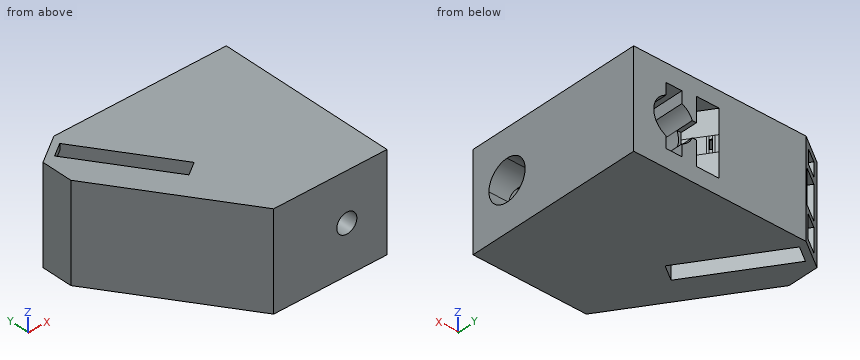
```python
from build123d import *
from build123d.topology import SkipClean

# Parameters (mm, degrees)
BOSS_EXTRUDE1_DEPTH     = 2.5
BOSS_EXTRUDE1_2_DEPTH   = 2.5
BOSS_EXTRUDE2_DEPTH     = 6.35
BOSS_EXTRUDE3_DEPTH     = 6.35
SKETCH4_R               = 3.175
CUT_EXTRUDE1_DEPTH      = 25.4
SKETCH5_R               = 1.5875
CUT_EXTRUDE2_DEPTH      = 25.4
CUT_EXTRUDE3_DEPTH      = 25.4
CUT_EXTRUDE4_REACH      = 43
CUT_EXTRUDE4_END_RADIUS = 3.175
CUT_EXTRUDE5_REACH      = 39.36
SKETCH8_W               = 2.54
SKETCH8_H               = 9.525
SKETCH9_W               = 0.508
SKETCH9_H               = 15.2
BOSS_EXTRUDE4_DEPTH     = 17
BOSS_EXTRUDE5_DEPTH     = 1.016
SKETCH11_W              = 1.176658287
SKETCH11_H              = 2.5
SKETCH11_W_2            = 2.433787944
SKETCH11_H_2            = 15.2
BOSS_EXTRUDE6_DEPTH     = 1.27
CUT_EXTRUDE6_DEPTH      = 38.864332241
BOSS_EXTRUDE7_START     = 2.54
BOSS_EXTRUDE7_DEPTH     = 2.54
BOSS_EXTRUDE8_DEPTH     = 2.54
BOSS_EXTRUDE9_DEPTH     = 0.508
BOSS_EXTRUDE10_DEPTH    = 0.508
CUT_EXTRUDE7_DEPTH      = 3.81
CUT_EXTRUDE8_DEPTH      = 3.81
BOSS_EXTRUDE11_DEPTH    = 3.81
SKETCH21_W              = 1.016
SKETCH21_H              = 1.016
SKETCH21_W_2            = 0.889
BOSS_EXTRUDE12_DEPTH    = 3.302
BOSS_EXTRUDE13_DEPTH    = 3.81


with BuildPart() as part:
    # Sketch1 → Boss-Extrude1 (new body)
    with BuildSketch(Plane.XY):
        Polygon((5.08, 0), (0, 0), (0, 19.141079028), (-1.033059908, 19.141079028), (-3.75575709, 23.125698967), (-8.376397661, 9.077684872), (-11.679025045, 6.820994294), (-21.26996, 20.857160675), (-22.86, 19.770683798), (-22.86, -3.81), (8.89, -3.81), (8.89, 24.384), (5.08, 24.384), align=None)
    extrude(amount=BOSS_EXTRUDE1_DEPTH)



with BuildPart() as body_2:
    # Sketch1 → Boss-Extrude1 2 (new body)
    with BuildSketch(Plane.XY):
        Polygon((-10.069369191, 23.749), (-4.328956497, 23.964566322), (-4.615556201, 24.384), (-16.108492032, 24.384), (-17.03780348, 23.749), align=None)
    extrude(amount=BOSS_EXTRUDE1_2_DEPTH)


with BuildPart() as part_1:
    add(part.part)

    add(body_2.part)  # Boss-Extrude2 merges body 2
    # Sketch2 → Boss-Extrude2 (add)
    with BuildSketch(Plane.XY.offset(2.5)):
        Polygon((-11.679025045, 6.820994294), (-21.26996, 20.857160675), (-22.86, 19.770683798), (-22.86, -3.81), (8.89, -3.81), (8.89, 24.384), (5.08, 24.384), (5.08, 0), (0, 0), (0, 19.141079028), (-1.033059908, 19.141079028), (-3.75575709, 23.125698967), (-8.376397661, 9.077684872), align=None)
        Polygon((-16.108492032, 24.384), (-18.00931945, 23.085161582), (-8.418384495, 9.048995201), (-8.376397661, 9.077684872), (-3.75575709, 23.125698967), (-1.033059908, 19.141079028), (0, 19.141079028), (0, 0), (5.08, 0), (5.08, 24.384), align=None)
    extrude(amount=BOSS_EXTRUDE2_DEPTH)

    # Sketch3 → Boss-Extrude3 (add)
    with BuildSketch(Plane(origin=(0, 0, 0), x_dir=(-1, 0, 0), z_dir=(0, 0, -1))):
        Polygon((-8.89, 24.384), (-8.89, -3.81), (22.86, -3.81), (22.86, 19.770683798), (21.26996, 20.857160675), (11.679025045, 6.820994294), (8.376397661, 9.077684872), (18.00931945, 23.085161582), (16.108492032, 24.384), align=None)
    extrude(amount=BOSS_EXTRUDE3_DEPTH)

    # Sketch4 → Cut-Extrude1 (cut)
    with BuildSketch(Plane(origin=(0, 24.384, 0), x_dir=(1, 0, 0), z_dir=(0, 1, 0))):
        with Locations(Location((2.54, -1.25, 0), (0, 0, 270))):
            Circle(SKETCH4_R)
    extrude(amount=-CUT_EXTRUDE1_DEPTH, mode=Mode.SUBTRACT)

    # Sketch5 → Cut-Extrude2 (cut)
    with BuildSketch(Plane(origin=(0, -1.016, 0), x_dir=(1, 0, 0), z_dir=(0, 1, 0))):
        with Locations(Location((2.54, -1.25, 0), (0, 0, 270))):
            Circle(SKETCH5_R)
    extrude(amount=-CUT_EXTRUDE2_DEPTH, mode=Mode.SUBTRACT)

    # Sketch6 → Cut-Extrude3 (cut)
    with BuildSketch(Plane.XY.offset(8.85)):
        Polygon((-22.86, 16.430904611), (-9.029357481, -3.81), (-22.86, -3.81), align=None)
    extrude(amount=-CUT_EXTRUDE3_DEPTH, mode=Mode.SUBTRACT)

    # Cut-Extrude4: up to this cylinder (the profile starts outside it)
    with SkipClean():  # the faces are left unmerged after this step: merging them gives an invalid solid
        cut_extrude4_end = Plane(origin=(2.54, 2.159, 1.25), z_dir=(0, 1, 0)) * Cylinder(CUT_EXTRUDE4_END_RADIUS, 96.045024, mode=Mode.PRIVATE)
        # Sketch7 → Cut-Extrude4 (cut, up to the surface)
        with BuildSketch(Plane(origin=(8.89, 0, 0), x_dir=(0, 0, -1), z_dir=(1, 0, 0)), mode=Mode.PRIVATE) as cut_extrude4_sk1:
            with BuildLine():
                ThreePointArc((1.925, 2.159), (-1.25, 5.334), (-4.425, 2.159))
                Line((-4.425, 2.159), (1.925, 2.159))
            make_face()
        cut_extrude4_tool1 = extrude(cut_extrude4_sk1.sketch, amount=-CUT_EXTRUDE4_REACH, mode=Mode.PRIVATE) - cut_extrude4_end
        add(cut_extrude4_tool1.solids().sort_by_distance((8.89, 3.506512, 1.25))[0], mode=Mode.SUBTRACT)
        # Sketch7 → Cut-Extrude4 (cut, up to the surface)
        with BuildSketch(Plane(origin=(8.89, 0, 0), x_dir=(0, 0, -1), z_dir=(1, 0, 0)), mode=Mode.PRIVATE) as cut_extrude4_sk2:
            with BuildLine():
                Line((1.925, 2.159), (-4.425, 2.159))
                ThreePointArc((-4.425, 2.159), (-3.49506403, -0.08606403), (-1.25, -1.016))
                ThreePointArc((-1.25, -1.016), (0.99506403, -0.08606403), (1.925, 2.159))
            make_face()
        cut_extrude4_tool2 = extrude(cut_extrude4_sk2.sketch, amount=-CUT_EXTRUDE4_REACH, mode=Mode.PRIVATE) - cut_extrude4_end
        add(cut_extrude4_tool2.solids().sort_by_distance((8.89, 0.811488, 1.25))[0], mode=Mode.SUBTRACT)
        # Sketch7 → Cut-Extrude4 (cut, up to the surface)
        with BuildSketch(Plane(origin=(8.89, 0, 0), x_dir=(0, 0, -1), z_dir=(1, 0, 0)), mode=Mode.PRIVATE) as cut_extrude4_sk3:
            with BuildLine():
                ThreePointArc((1.925, 2.159), (-1.25, 5.334), (-4.425, 2.159))
                Line((-4.425, 2.159), (1.925, 2.159))
            make_face()
        cut_extrude4_tool3 = extrude(cut_extrude4_sk3.sketch, amount=-CUT_EXTRUDE4_REACH, mode=Mode.PRIVATE) - cut_extrude4_end
        add(cut_extrude4_tool3.solids().sort_by_distance((8.89, 3.506512, 1.25))[0], mode=Mode.SUBTRACT)
        # Sketch7 → Cut-Extrude4 (cut, up to the surface)
        with BuildSketch(Plane(origin=(8.89, 0, 0), x_dir=(0, 0, -1), z_dir=(1, 0, 0)), mode=Mode.PRIVATE) as cut_extrude4_sk4:
            with BuildLine():
                Line((1.925, 2.159), (-4.425, 2.159))
                ThreePointArc((-4.425, 2.159), (-3.49506403, -0.08606403), (-1.25, -1.016))
                ThreePointArc((-1.25, -1.016), (0.99506403, -0.08606403), (1.925, 2.159))
            make_face()
        cut_extrude4_tool4 = extrude(cut_extrude4_sk4.sketch, amount=-CUT_EXTRUDE4_REACH, mode=Mode.PRIVATE) - cut_extrude4_end
        add(cut_extrude4_tool4.solids().sort_by_distance((8.89, 0.811488, 1.25))[0], mode=Mode.SUBTRACT)

    # Cut-Extrude5: up to this face of the body (flat: up to its plane)
    cut_extrude5_end = Plane(part_1.part.faces().sort_by_distance((4.72156403, -1.016, 3.43156403))[0])
    # Sketch8 → Cut-Extrude5 (cut, up to the picked face)
    with BuildSketch(Plane(origin=(0, 24.384, 0), x_dir=(1, 0, 0), z_dir=(0, 1, 0)), mode=Mode.PRIVATE) as cut_extrude5_sk1:
        with Locations((2.54, -1.25)):
            Rectangle(SKETCH8_W, SKETCH8_H)
    cut_extrude5_tool1 = split(extrude(cut_extrude5_sk1.sketch, amount=-CUT_EXTRUDE5_REACH, mode=Mode.PRIVATE), bisect_by=cut_extrude5_end, keep=Keep.BOTH, mode=Mode.PRIVATE)
    add(cut_extrude5_tool1.solids().sort_by(Axis((2.54, 24.384, 1.25), (0, -1, 0)))[0], mode=Mode.SUBTRACT)

    # Sketch9 → Boss-Extrude4 (add)
    with BuildSketch(Plane(origin=(-6.894633763, 10.090176515, 0), x_dir=(0.825656845959394, 0.5641726444275594, 0), z_dir=(-0.5641726444275594, 0.825656845959394, 0))):
        with Locations((-5.540648594, -1.25)):
            Rectangle(SKETCH9_W, SKETCH9_H)
        Polygon((-1.794648594, 6.35), (-2.302648594, 6.35), (-2.302648594, 1.6202), (-3.623501238, 1.6202), (-3.623501238, 0.7312), (-1.794648594, 0.7312), align=None)
        Polygon((-1.845501238, -8.85), (-1.845501238, -4.6028), (-3.572648594, -4.6028), (-3.572648594, -5.6188), (-2.683648594, -5.6188), (-2.683648594, -8.85), align=None)
    extrude(amount=BOSS_EXTRUDE4_DEPTH)

    # Sketch10 → Boss-Extrude5 (add)
    with BuildSketch(Plane(origin=(-6.894633763, 10.090176515, 0), x_dir=(0.8256568459593948, 0.5641726444275585, 0), z_dir=(-0.5641726444275585, 0.8256568459593948, 0))):
        Polygon((-5.286648594, -8.85), (-2.683648594, -8.85), (-2.683648594, -5.6188), (-3.572648594, -5.6188), (-3.572648594, -4.6028), (-1.845501238, -4.6028), (-1.845501238, -2.5), (-1.794648594, -2.5), (-1.794648594, 0), (-1.794648594, 0.7312), (-3.623501238, 0.7312), (-3.623501238, 1.6202), (-2.302648594, 1.6202), (-2.302648594, 6.35), (-5.286648594, 6.35), align=None)
    extrude(amount=BOSS_EXTRUDE5_DEPTH)

    # Sketch11 → Boss-Extrude6 (add)
    with BuildSketch(Plane(origin=(-16.485568719, 24.126342896, 0), x_dir=(0.8256568459593935, 0.5641726444275603, 0), z_dir=(-0.5641726444275603, 0.8256568459593935, 0))):
        with Locations((-1.257172095, -1.25)):
            Rectangle(SKETCH11_W, SKETCH11_H)
        Polygon((-3.623501238, 1.6202), (-3.623501238, 0.7312), (-1.845501238, 0.7312), (-1.845501238, 0), (-0.668842951, 0), (-0.668842951, -2.5), (-1.845501238, -2.5), (-1.845501238, -4.6028), (-3.572648594, -4.6028), (-3.572648594, -5.6188), (-2.683648594, -5.6188), (-2.683648594, -8.85), (0.456699038, -8.85), (0.456699038, 6.35), (-2.302648594, 6.35), (-2.302648594, 1.6202), align=None)
        with Locations((-6.503542566, -1.25)):
            Rectangle(SKETCH11_W_2, SKETCH11_H_2)
    extrude(amount=BOSS_EXTRUDE6_DEPTH)

    # Sketch12 → Cut-Extrude6 (cut, through all)
    with BuildSketch(Plane.XY.offset(8.85)):
        Polygon((-16.108492032, 24.384), (-18.359576008, 24.384), (-16.82499129, 25.432584194), align=None)
        Polygon((-22.86, 19.770683798), (-22.86, 21.308853083), (-23.576499258, 20.819267993), align=None)
    extrude(amount=-CUT_EXTRUDE6_DEPTH, mode=Mode.SUBTRACT)

    # Sketch13 → Boss-Extrude7 (add)
    with BuildSketch(Plane(origin=(0, 19.141079028, 0), x_dir=(1, 0, 0), z_dir=(0, 1, 0)).offset(BOSS_EXTRUDE7_START)):
        with BuildLine():
            Line((-0.378582704, 0), (-1.033059908, 0))
            Line((-1.033059908, 0), (-1.033059908, -2.5))
            Line((-1.033059908, -2.5), (-0.378582704, -2.5))
            ThreePointArc((-0.378582704, -2.5), (-0.635, -1.25), (-0.378582704, 0))
        make_face()
    extrude(amount=-BOSS_EXTRUDE7_DEPTH)

    # Sketch15 → Boss-Extrude8 (add)
    with BuildSketch(Plane.XY):
        Polygon((-4.156996675, 23.712906116), (-4.328956497, 23.964566322), (-4.538912798, 23.956681957), (-4.303798462, 23.612596219), align=None)
        Polygon((-3.75575709, 23.125698967), (-3.927716912, 23.377359173), (-4.0745187, 23.277049277), (-3.825732396, 22.912954853), align=None)
    extrude(amount=BOSS_EXTRUDE8_DEPTH)

    # Sketch16 → Boss-Extrude9 (add)
    with BuildSketch(Plane.XY):
        Polygon((-4.0745187, 23.277049277), (-4.303798462, 23.612596219), (-4.156996675, 23.712906116), (-3.927716912, 23.377359173), align=None)
    extrude(amount=BOSS_EXTRUDE9_DEPTH)

    # Sketch17 → Boss-Extrude10 (add)
    with BuildSketch(Plane(origin=(0, 0, 2.5), x_dir=(-1, 0, 0), z_dir=(0, 0, -1))):
        Polygon((4.0745187, 23.277049277), (4.303798462, 23.612596219), (4.156996675, 23.712906116), (3.927716912, 23.377359173), align=None)
    extrude(amount=BOSS_EXTRUDE10_DEPTH)

    # Sketch18 → Cut-Extrude7 (cut)
    with BuildSketch(Plane(origin=(0, 0, 2.5), x_dir=(-1, 0, 0), z_dir=(0, 0, -1))):
        Polygon((1.033059908, 24.384), (1.033059908, 21.681079028), (1.033059908, 19.141079028), (4.615556201, 24.384), align=None)
    extrude(amount=-CUT_EXTRUDE7_DEPTH, mode=Mode.SUBTRACT)

    # Sketch19 → Cut-Extrude8 (cut)
    with BuildSketch(Plane.XY):
        Polygon((-1.033059908, 19.141079028), (-1.033059908, 21.681079028), (-1.033059908, 24.384), (-4.615556201, 24.384), align=None)
    extrude(amount=-CUT_EXTRUDE8_DEPTH, mode=Mode.SUBTRACT)

    # Sketch20 → Boss-Extrude11 (add)
    with BuildSketch(Plane.XY):
        Polygon((-10.069369191, 23.749), (-4.303798462, 23.612596219), (-4.538912798, 23.956681957), align=None)
    extrude(amount=BOSS_EXTRUDE11_DEPTH)

    # Sketch21 → Boss-Extrude12 (add)
    with BuildSketch(Plane(origin=(-4.364957604, -2.982582517, 0), x_dir=(0, 0, -1), z_dir=(0.8256568459593941, 0.5641726444275595, 0))):
        with Locations((5.842, 29.982787079)):
            Rectangle(SKETCH21_W, SKETCH21_H)
        with Locations((1.1757, 29.982787079)):
            Rectangle(SKETCH21_W_2, SKETCH21_H)
        with Locations((-5.1108, 29.982787079)):
            Rectangle(SKETCH21_W, SKETCH21_H)
        with Locations((-8.342, 29.982787079)):
            Rectangle(SKETCH21_W, SKETCH21_H)
    extrude(amount=BOSS_EXTRUDE12_DEPTH)

    # Sketch22 → Boss-Extrude13 (add)
    with BuildSketch(Plane.XY):
        Polygon((-3.825732396, 22.912954853), (-4.0745187, 23.277049277), (-4.222544103, 21.706538478), align=None)
    extrude(amount=BOSS_EXTRUDE13_DEPTH)


solid = part_1.part
```
Geometry: final body of the model. Coordinates: model frame, mm. Coordinates: 2 decimals unless noted, no trailing zeros. Order: outer loops, then holes, each group sorted by start corner. A loop starts at its lowest first (then second) coordinate and runs counter-clockwise, first axis right, second up. Notation, with made-up numbers: (25.25, 47) -> (52.25, 47) arc R25 ccw to (52.25, 74) -> close; hole circle Ø5 at (14, 7). An arc over 180 degrees is marked (long way). Answer in a Markdown table with one row per item.
Item 1: Ray query, L1, parallel to Z at x = 1.5, y = 18.5; L2, parallel to X at y = 18.25, z = 5.25; L3, parallel to X at y = 8.75, z = -2.5. Return the intervals inside material, ascending.
Return value:
| item | result |
|---|---|
| L1 | z = -6.35 to -3.51, 6.01 to 8.85 |
| L2 | x = -22.86 to -18.87, -16.8 to 1.27, 3.81 to 8.89 |
| L3 | x = -17.61 to -12.38, -10.66 to 1.27, 3.81 to 8.89 |
Item 2: Section C-C on x = -13.5. Output: boundary loops of the cut face in (y, z), plus the area to 3 significant figures.
Return value:
| item | result |
|---|---|
| outline | (2.73, -6.35) -> (10.39, -6.35) -> (10.39, 8.85) -> (2.73, 8.85) -> close; (13.33, -1.62) -> (15.68, -1.62) -> (15.68, -6.35) -> (24.38, -6.35) -> (24.38, 8.85) -> (15, 8.85) -> (15, 5.62) -> (13.42, 5.62) -> (13.42, 4.6) -> (16.49, 4.6) -> (16.49, 2.5) -> (23.75, 2.5) -> (23.75, 0) -> (16.53, 0) -> (16.53, -0.73) -> (13.33, -0.73) -> close |
| area | 233 mm² |
Item 3: Section A-A on x = 2.54. Output: boundary loops of the cut face in (y, z), plus the area to 3 significant figures.
Return value:
| item | result |
|---|---|
| outline | (-3.81, -6.35) -> (24.38, -6.35) -> (24.38, -3.51) -> (-1.02, -3.51) -> (-1.02, -0.34) -> (-3.81, -0.34) -> close; (-3.81, 2.84) -> (-1.02, 2.84) -> (-1.02, 6.01) -> (24.38, 6.01) -> (24.38, 8.85) -> (-3.81, 8.85) -> close |
| area | 178 mm² |
Item 4: Contact query for flat-ended pins moving along their axis: P1, Ø1, axis at y = 13.5, z = 4.5, coming from the -X side; P2, Ø8, axis at y = 2.5, z = 3, coming from the -X side; P3, Ø0.9, axis at y = 6.5, z = -2.5, coming from the -X side. Output: stop coordinate, or through.
Return value:
| item | result |
|---|---|
| P1 | stops at x = -21.2 |
| P2 | stops at x = -16.07 |
| P3 | stops at x = -16.38 |
Item 5: Section B-B on x = -7.5. Output: boundary loops of the cut face in (y, z).
Return value:
| item | result |
|---|---|
| outline | (-3.81, -6.35) -> (24.38, -6.35) -> (24.38, 8.85) -> (-3.81, 8.85) -> close; hole (11.74, 0) -> (23.69, 0) -> (23.69, 2.5) -> (11.74, 2.5) -> close |
